Work out the finished part from the listing and answer in its coordinate system (mm). Face numbers are marked on the shaded views. A direction names the side the tool comes from. Coordinates: 2 decimals unless noted, no trailing zeros. Loops run counter-clockwise (first coordinate to the right, second up) from the corner with the lowest first, then second, coordinate; pieces in that order, holes last. Notation, with made-up numbers: (-8.75, 34.5) -> (39.25, 34.5) arc R21 ccw to (39.25, 59.5) -> close; hole circle Ø11 at (11, 25.25). An arc over 180 degrees is marked (long way). Answer as CSV lines item,"result".
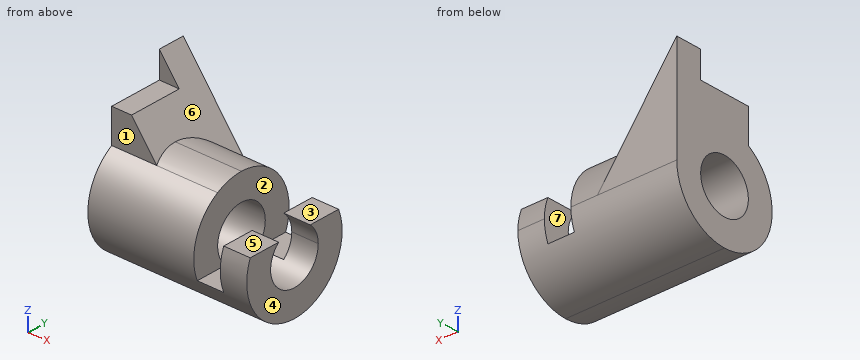
```python
from build123d import *

# Parameters (mm, degrees)
F1_DEPTH  = 25.4
F3_DEPTH  = 76.201
F5_DEPTH  = 76.201
F7_DEPTH  = 31.75
F10_R     = 12.7
F11_DEPTH = 76.201
F13_DEPTH = 12.7
F15_DEPTH = 12.7


with BuildPart() as f1:
    # F0 (on Front) → F1 (new body, symmetric)
    with BuildSketch(Plane.XZ):
        Polygon((0, 47.625), (0, 0), (76.2, 0), (76.2, 34.925), (63.5, 34.925), (63.5, 15.875), (50.8, 15.875), (50.8, 50.8), (19.05, 50.8), (21.43125, 47.625), align=None)
        Polygon((0, 76.2), (0, 47.625), (21.43125, 47.625), (19.05, 50.8), align=None)
    extrude(amount=F1_DEPTH, both=True)

    # F2 (on face) → F3 (cut, through all)
    with BuildSketch(Plane.YZ.offset(76.2)):
        with BuildLine():
            Line((-25.4, 0), (-1.82e-08, 0))
            ThreePointArc((-1.82e-08, 0), (-17.9605122486, 7.4394877643), (-25.4, 25.4))
            Line((-25.4, 25.4), (-25.4, 0))
        make_face()
        with BuildLine():
            Line((25.4, 0), (25.4, 25.4))
            ThreePointArc((25.4, 25.4), (17.9605122357, 7.4394877514), (-1.82e-08, 0))
            Line((-1.82e-08, 0), (25.4, 0))
        make_face()
    extrude(amount=-F3_DEPTH, mode=Mode.SUBTRACT)

    # F4 (on Right) → F5 (cut, through all)
    with BuildSketch(Plane.YZ):
        with BuildLine():
            Line((12.7, 63.5), (12.7, 76.2))
            Line((12.7, 76.2), (-25.4, 76.2))
            Line((-25.4, 76.2), (-25.4, 25.4))
            ThreePointArc((-25.4, 25.4), (-21.9970452561, 38.1), (-12.7, 47.3970452561))
            Line((-12.7, 47.3970452561), (-12.7, 63.5))
            Line((-12.7, 63.5), (12.7, 63.5))
        make_face()
    extrude(amount=F5_DEPTH, mode=Mode.SUBTRACT)

    # F6 (on face) → F7 (cut)
    with BuildSketch(Plane.YZ.offset(50.8)):
        with BuildLine():
            ThreePointArc((6.88e-08, 50.8), (17.9605122665, 43.3605122178), (25.4, 25.4))
            Line((25.4, 25.4), (25.4, 50.8))
            Line((25.4, 50.8), (6.88e-08, 50.8))
        make_face()
        with BuildLine():
            ThreePointArc((-12.7, 47.3970452561), (-6.5740037124, 49.9345159966), (6.88e-08, 50.8))
            Line((6.88e-08, 50.8), (-12.7, 50.8))
            Line((-12.7, 50.8), (-12.7, 47.3970452561))
        make_face()
    extrude(amount=-F7_DEPTH, mode=Mode.SUBTRACT)

    # F8 (on face) → F9 (join, up to the next surface of F1)
    with BuildSketch(Plane(origin=(0, 25.4, 0), x_dir=(-1, 0, 0), z_dir=(0, 1, 0))):
        Polygon((-38.1, 25.4), (-19.05, 25.4), (-19.05, 50.8), align=None)
    extrude(until=Until.NEXT, dir=(0, -1, 0))

    # F10 (on face) → F11 (cut, through all)
    with BuildSketch(Plane.YZ.offset(76.2)):
        with Locations((0, 25.4)):
            Circle(F10_R)
    extrude(amount=-F11_DEPTH, mode=Mode.SUBTRACT)

    # F12 (on face) → F13 (cut)
    with BuildSketch(Plane.YZ.offset(76.2)):
        with BuildLine():
            ThreePointArc((23.5464301965, 34.925), (24.9323016085, 30.2518384664), (25.4, 25.4))
            Line((25.4, 25.4), (25.4, 34.925))
            Line((25.4, 34.925), (23.5464301965, 34.925))
        make_face()
    extrude(amount=-F13_DEPTH, mode=Mode.SUBTRACT)

    # F14 (on face) → F15 (join)
    with BuildSketch(Plane.XZ.offset(12.7)):
        Polygon((0, 63.5), (0, 47.3970452561), (21.6022160579, 47.3970452561), (9.525, 63.5), align=None)
    extrude(amount=-F15_DEPTH)


solid = f1.part
```
(1) For a pull along X with two mould halves and no side action, classify the marked faces 5, 6 and 7 as pulls with the +X half, pulls with the -X half, needs draft (parallel to the pull), parting line crosses it, or undercut.
Computed values:
face 5,"needs draft"
face 6,"pulls with the +X half"
face 7,"undercut"
(2) A cutting plane is placed at B-B, the plane x = 10.5. Write down the section's boundary in (y, z).
Computed values:
outline,"(-12.7, 47.4) arc R25.4 ccw (long way) to (25.4, 25.4) -> (25.4, 62.2) -> (-12.7, 62.2) -> close; hole circle Ø25.4 at (0, 25.4)"
(3) A cutting plane is placed at C-C, the plane y = -10.5. Write down the section's boundary in (x, z) (3 decimals), and give its area (3 significant figures).
Computed values:
outline,"(0, 2.272) -> (76.2, 2.272) -> (76.2, 18.256) -> (63.5, 18.256) -> (63.5, 15.875) -> (50.8, 15.875) -> (50.8, 18.256) -> (0, 18.256) -> close; (0, 32.544) -> (50.8, 32.544) -> (50.8, 48.528) -> (20.754, 48.528) -> (9.525, 63.5) -> (0, 63.5) -> close; (63.5, 32.544) -> (76.2, 32.544) -> (76.2, 34.925) -> (63.5, 34.925) -> close"
area,"2,260 mm2"
(4) Flat-ended cylindrical pins translate along their axes: pin 1 Ø20.5 at (y, z) = (0, 25.4) entering from +X; pin 2 Ø1.5 at (y, z) = (3.5, 53.5) entering from +X; pin 3 Ø8 at (x, z) = (17, 60) entering from -Y; pin 4 Ø5 at (x, z) = (3.5, 68) entering from -Y. Find the tip coordinate at first contact, or state that the pin passes through.
Computed values:
pin 1,"through"
pin 2,"x = 17.59"
pin 3,"y = -12.7"
pin 4,"y = 12.7"
(5) A cutting plane is placed at D-D, the plane x = 58. Write down the section's boundary in (y, z) (3 decimals).
Computed values:
outline,"(-23.546, 15.875) arc R25.4 ccw to (23.546, 15.875) -> (8.4, 15.875) arc R12.7 cw to (-8.4, 15.875) -> close"
(6) A cutting plane is placed at A-A, the plane z = 14. Write down the section's boundary in (x, y), and give its area (3 significant figures).
Computed values:
outline,"(0, -22.7) -> (76.2, -22.7) -> (76.2, -5.6) -> (0, -5.6) -> close; (0, 5.6) -> (76.2, 5.6) -> (76.2, 22.7) -> (0, 22.7) -> close"
area,"2,610 mm2"
(7) Which of the six approach directions +Z, -Z, +X, -X, +Y, -Y give full straight-line access (tool end or side, diameter ignored) to the marked faces 1, 2, 3 and 4?
Computed values:
face 1,"+Z, +X, -X, -Y"
face 2,"+Z, +Y, -Y"
face 3,"+Z, +X, +Y, -Y"
face 4,"+Z, -Z, +X, +Y, -Y"
(8) Consider line 1 along Y through (x, z) = (21, 25.4); line 2 along X through (y, z) = (-16, 27); line 3 along Z through (x, y) = (31, -0.5). Determine where each line is inside the solid, lowest interval first.
Computed values:
line 1,"-25.4 to -12.7, 12.7 to 25.4"
line 2,"0 to 50.8, 63.5 to 76.2"
line 3,"0 to 12.71, 38.09 to 50.8"
